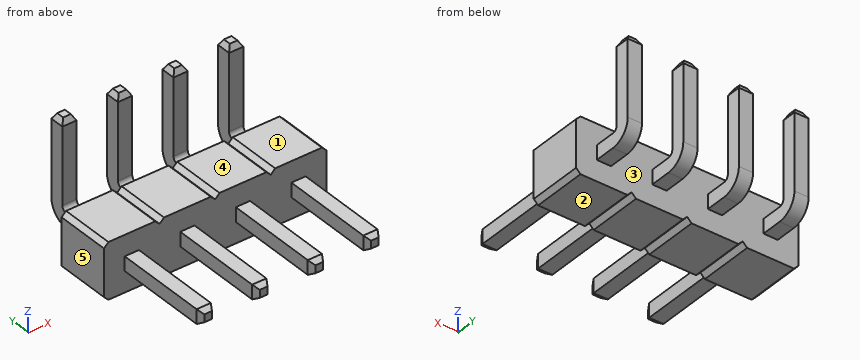
from build123d import *

# Parameters (mm, degrees)
BOSS_EXTRUDE1_DEPTH = 2.5
SKETCH3_W           = 0.65
SKETCH3_H           = 0.65
BOSS_EXTRUDE2_DEPTH = 6
SKETCH4_W           = 0.65
SKETCH4_H           = 0.65
CHAMFER3_SIZE       = 0.15
CHAMFER3_SIZE2      = 0.259807621
CHAMFER2_SIZE       = 0.15
CHAMFER2_SIZE2      = 0.259807621
LPATTERN2_START     = -5.08
LPATTERN2_OUTLINE_W = 2.5
LPATTERN2_OUTLINE_H = 2.54
LPATTERN2_DEPTH     = 7.62
LPATTERN2_START_2   = -4.135
LPATTERN2_2_DEPTH   = 0.65
LPATTERN2_START_3   = -1.595
LPATTERN2_3_DEPTH   = 0.65
LPATTERN2_START_4   = 0.945
LPATTERN2_4_DEPTH   = 0.65
LPATTERN2_START_5   = -4.240192379
LPATTERN2_5_DEPTH   = 9.240192379
LPATTERN2_START_6   = -1
LPATTERN2_6_DEPTH   = 2


with BuildPart() as part:
    # Sketch1 → Boss-Extrude1 (new body)
    with BuildSketch(Plane(origin=(0, 0, 0), x_dir=(1, 0, 0), z_dir=(0, 1, 0))):
        Polygon((-7.42, 1.27), (-7.62, 1.07), (-7.62, -1.07), (-7.42, -1.27), (-5.28, -1.27), (-5.08, -1.07), (-5.08, 1.07), (-5.28, 1.27), align=None)
    extrude(amount=BOSS_EXTRUDE1_DEPTH)

    # Sketch3 → Boss-Extrude2 (add)
    with BuildSketch(Plane(origin=(0, -4.5, 0), x_dir=(1, 0, 0), z_dir=(0, 1, 0))):
        with Locations((-6.35, 0)):
            Rectangle(SKETCH3_W, SKETCH3_H)
    extrude(amount=BOSS_EXTRUDE2_DEPTH)

    # Sweep1: sweep along a path in Sketch5
    with BuildLine(Plane.ZY.offset(6.35)) as sweep1_path:
        Line((0, 2.5), (0, 3.45))
        ThreePointArc((0, 3.45), (0.16109127, 3.83890873), (0.55, 4))
        Line((0.55, 4), (4.27, 4))
    # Sketch4 → Sweep1 (sweep)
    with BuildSketch(Plane(origin=(0, 2.5, 0), x_dir=(1, 0, 0), z_dir=(0, 1, 0))):
        with Locations((-6.35, 0)):
            Rectangle(SKETCH4_W, SKETCH4_H)
    sweep(path=sweep1_path.line)

    # Chamfer3
    chamfer3_edges = [part.edges().sort_by_distance(p)[0] for p in [
        (-6.675, 4, 4.27),
        (-6.35, 3.675, 4.27),
        (-6.025, 4, 4.27),
        (-6.35, 4.325, 4.27),
    ]]
    chamfer3_side = [part.faces().sort_by_distance(p)[0] for p in [
        (-6.35, 4, 4.27),
    ]]
    chamfer(chamfer3_edges, length=CHAMFER3_SIZE, length2=CHAMFER3_SIZE2, reference=chamfer3_side[0])

    # Chamfer2
    chamfer2_edges = [part.edges().sort_by_distance(p)[0] for p in [
        (-6.025, -4.5, 0),
        (-6.35, -4.5, -0.325),
        (-6.675, -4.5, 0),
        (-6.35, -4.5, 0.325),
    ]]
    chamfer2_side = [part.faces().sort_by_distance(p)[0] for p in [
        (-6.35, -4.5, 0),
    ]]
    chamfer(chamfer2_edges, length=CHAMFER2_SIZE, length2=CHAMFER2_SIZE2, reference=chamfer2_side[0])

    # LPattern2: read off the stored shape, not the designer's step
    # LPattern2 outline → LPattern2 (add)
    with BuildSketch(Plane.YZ.offset(LPATTERN2_START)):
        with Locations((1.25, 0)):
            Rectangle(LPATTERN2_OUTLINE_W, LPATTERN2_OUTLINE_H)
    extrude(amount=LPATTERN2_DEPTH)

    # LPattern2 2 outline → LPattern2 2 (add)
    with BuildSketch(Plane.YZ.offset(LPATTERN2_START_2)):
        Polygon((0, -0.325), (0, 0.325), (-4.240192379, 0.325), (-4.5, 0.175), (-4.5, -0.175), (-4.240192379, -0.325), align=None)
        with BuildLine():
            Line((3.45, 0.325), (2.5, 0.325))
            Line((2.5, 0.325), (2.5, -0.325))
            Line((2.5, -0.325), (3.45, -0.325))
            ThreePointArc((3.45, -0.325), (4.068718434, -0.068718434), (4.325, 0.55))
            Line((4.325, 0.55), (4.325, 4.010192379))
            Line((4.325, 4.010192379), (4.175, 4.27))
            Line((4.175, 4.27), (3.825, 4.27))
            Line((3.825, 4.27), (3.675, 4.010192379))
            Line((3.675, 4.010192379), (3.675, 0.55))
            ThreePointArc((3.675, 0.55), (3.609099026, 0.390900974), (3.45, 0.325))
        make_face()
    extrude(amount=LPATTERN2_2_DEPTH)

    # LPattern2 3 outline → LPattern2 3 (add)
    with BuildSketch(Plane.YZ.offset(LPATTERN2_START_3)):
        Polygon((0, -0.325), (0, 0.325), (-4.240192379, 0.325), (-4.5, 0.175), (-4.5, -0.175), (-4.240192379, -0.325), align=None)
        with BuildLine():
            Line((3.45, 0.325), (2.5, 0.325))
            Line((2.5, 0.325), (2.5, -0.325))
            Line((2.5, -0.325), (3.45, -0.325))
            ThreePointArc((3.45, -0.325), (4.068718434, -0.068718434), (4.325, 0.55))
            Line((4.325, 0.55), (4.325, 4.010192379))
            Line((4.325, 4.010192379), (4.175, 4.27))
            Line((4.175, 4.27), (3.825, 4.27))
            Line((3.825, 4.27), (3.675, 4.010192379))
            Line((3.675, 4.010192379), (3.675, 0.55))
            ThreePointArc((3.675, 0.55), (3.609099026, 0.390900974), (3.45, 0.325))
        make_face()
    extrude(amount=LPATTERN2_3_DEPTH)

    # LPattern2 4 outline → LPattern2 4 (add)
    with BuildSketch(Plane.YZ.offset(LPATTERN2_START_4)):
        Polygon((0, -0.325), (0, 0.325), (-4.240192379, 0.325), (-4.5, 0.175), (-4.5, -0.175), (-4.240192379, -0.325), align=None)
        with BuildLine():
            Line((3.45, 0.325), (2.5, 0.325))
            Line((2.5, 0.325), (2.5, -0.325))
            Line((2.5, -0.325), (3.45, -0.325))
            ThreePointArc((3.45, -0.325), (4.068718434, -0.068718434), (4.325, 0.55))
            Line((4.325, 0.55), (4.325, 4.010192379))
            Line((4.325, 4.010192379), (4.175, 4.27))
            Line((4.175, 4.27), (3.825, 4.27))
            Line((3.825, 4.27), (3.675, 4.010192379))
            Line((3.675, 4.010192379), (3.675, 0.55))
            ThreePointArc((3.675, 0.55), (3.609099026, 0.390900974), (3.45, 0.325))
        make_face()
    extrude(amount=LPATTERN2_4_DEPTH)

    # LPattern2 5 outline → LPattern2 5 (cut)
    with BuildSketch(Plane(origin=(0, 0, 0), x_dir=(1, 0, 0), z_dir=(0, 1, 0)).offset(LPATTERN2_START_5)):
        Polygon((-5.08, 1.27), (-5.08, 1.07), (-4.88, 1.27), align=None)
        Polygon((-5.08, -1.27), (-4.88, -1.27), (-5.08, -1.07), align=None)
        Polygon((-2.74, -1.27), (-2.34, -1.27), (-2.54, -1.07), align=None)
        Polygon((-0.2, -1.27), (0.2, -1.27), (0, -1.07), align=None)
        Polygon((2.54, -1.27), (2.54, -1.07), (2.34, -1.27), align=None)
        Polygon((2.54, 1.27), (2.34, 1.27), (2.54, 1.07), align=None)
        Polygon((0.2, 1.27), (-0.2, 1.27), (0, 1.07), align=None)
        Polygon((-2.34, 1.27), (-2.74, 1.27), (-2.54, 1.07), align=None)
        Polygon((1.595, -4.27), (1.595, -4.010192379), (1.445, -4.27), align=None)
        Polygon((1.095, -4.27), (0.945, -4.010192379), (0.945, -4.27), align=None)
        Polygon((-0.945, -4.27), (-0.945, -4.010192379), (-1.095, -4.27), align=None)
        Polygon((-1.445, -4.27), (-1.595, -4.010192379), (-1.595, -4.27), align=None)
        Polygon((-3.485, -4.27), (-3.485, -4.010192379), (-3.635, -4.27), align=None)
        Polygon((-3.985, -4.27), (-4.135, -4.010192379), (-4.135, -4.27), align=None)
    extrude(amount=LPATTERN2_5_DEPTH, mode=Mode.SUBTRACT)

    # LPattern2 6 outline → LPattern2 6 (cut)
    with BuildSketch(Plane.XY.offset(LPATTERN2_START_6)):
        Polygon((-3.485, -4.5), (-3.485, -4.240192379), (-3.635, -4.5), align=None)
        Polygon((-4.135, -4.5), (-3.985, -4.5), (-4.135, -4.240192379), align=None)
        Polygon((-0.945, -4.5), (-0.945, -4.240192379), (-1.095, -4.5), align=None)
        Polygon((-1.595, -4.5), (-1.445, -4.5), (-1.595, -4.240192379), align=None)
        Polygon((1.595, -4.5), (1.595, -4.240192379), (1.445, -4.5), align=None)
        Polygon((0.945, -4.5), (1.095, -4.5), (0.945, -4.240192379), align=None)
    extrude(amount=LPATTERN2_6_DEPTH, mode=Mode.SUBTRACT)


solid = part.part
Geometry: final body of the model. Coordinates: model frame, mm. Face numbers are marked on the shaded views. A direction names the side the tool comes from. Give positions to 0.01 mm unless a question says otherwise; leave off trailing zeros. Write each loop counter-clockwise with the first axis right and the second up, starting at its lowest first coordinate (ties: lowest second). Pieces come first, ordered by that corner, then holes.
(1) Mould query, pull axis X, two halves, no side actions, for the marked faces 3, 4 and 5. Classes: released by +X, released by -X, zero draft, split by the parting line, or undercut.
(2) Cut plane A-A, the plane y = -0.25. Return loops of the section in (x, z) (3 decimals).
(3) Ray query, line 1 (Y direction, x = -1, z = 0.65) (3 decimals); line 2 (X direction, y = -1.5, z = 0.2) (3 decimals); line 3 (Y direction, x = -1, z = 2.35) (3 decimals). Return the intervals inside material, ascending.
(4) Cut plane C-C, the plane z = 2.85. Return loops of the section in (x, y) (3 decimals), then the cut area to 3 significant figures.
(5) Cut plane B-B, the plane z = 0.75. Return loops of the section in (x, y) (3 decimals).
(6) Cut plane D-D, the plane y = 1.25. Return loops of the section in (x, z).
(7) First-contact query: P1, Ø0.5, axis at x = -1.5, y = -1, coming from the -Z side (3 decimals); P2, Ø1, axis at y = -2.5, z = -0.5, coming from the +X side (3 decimals); P3, Ø0.7, axis at x = 1.5, y = -1, coming from the +Z side (3 decimals). Flat tips, straight axial feed; report the tip coordinate or a pass-through.
(8) Access query for the marked faces 1 and 2. Directions: +Z, -Z, +X, -X, +Y, -Y. A direction counts if a zero-diameter tool reaches every point of the face in a straight line with its end or side. Return the directions, or none.
Values follow:
1. face 3: undercut
1. face 4: zero draft
1. face 5: released by -X
2. outline: (-6.675, -0.325) - (-6.025, -0.325) - (-6.025, 0.325) - (-6.675, 0.325) - close; (-4.135, -0.325) - (-3.485, -0.325) - (-3.485, 0.325) - (-4.135, 0.325) - close; (-1.595, -0.325) - (-0.945, -0.325) - (-0.945, 0.325) - (-1.595, 0.325) - close; (0.945, -0.325) - (1.595, -0.325) - (1.595, 0.325) - (0.945, 0.325) - close
3. line 1: y = 0 to 2.5, 3.675 to 4.325
3. line 2: x = -6.675 to -6.025, -4.135 to -3.485, -1.595 to -0.945, 0.945 to 1.595
3. line 3: y = 3.675 to 4.325
4. outline: (-6.675, 3.675) - (-6.025, 3.675) - (-6.025, 4.325) - (-6.675, 4.325) - close; (-4.135, 3.675) - (-3.485, 3.675) - (-3.485, 4.325) - (-4.135, 4.325) - close; (-1.595, 3.675) - (-0.945, 3.675) - (-0.945, 4.325) - (-1.595, 4.325) - close; (0.945, 3.675) - (1.595, 3.675) - (1.595, 4.325) - (0.945, 4.325) - close
4. area: 1.69 mm2
5. outline: (-7.62, 0) - (2.54, 0) - (2.54, 2.5) - (-7.62, 2.5) - close; (-6.675, 3.675) - (-6.025, 3.675) - (-6.025, 4.325) - (-6.675, 4.325) - close; (-4.135, 3.675) - (-3.485, 3.675) - (-3.485, 4.325) - (-4.135, 4.325) - close; (-1.595, 3.675) - (-0.945, 3.675) - (-0.945, 4.325) - (-1.595, 4.325) - close; (0.945, 3.675) - (1.595, 3.675) - (1.595, 4.325) - (0.945, 4.325) - close
6. outline: (-7.62, -1.07) - (-7.42, -1.27) - (-5.28, -1.27) - (-5.08, -1.07) - (-4.88, -1.27) - (-2.74, -1.27) - (-2.54, -1.07) - (-2.34, -1.27) - (-0.2, -1.27) - (0, -1.07) - (0.2, -1.27) - (2.34, -1.27) - (2.54, -1.07) - (2.54, 1.07) - (2.34, 1.27) - (0.2, 1.27) - (0, 1.07) - (-0.2, 1.27) - (-2.34, 1.27) - (-2.54, 1.07) - (-2.74, 1.27) - (-4.88, 1.27) - (-5.08, 1.07) - (-5.28, 1.27) - (-7.42, 1.27) - (-7.62, 1.07) - close
7. P1: stops at z = -0.325
7. P2: stops at x = 1.595
7. P3: stops at z = 0.325
8. face 1: +Z, +X, -X, -Y
8. face 2: -Z, +X, -X, +Y, -Y
